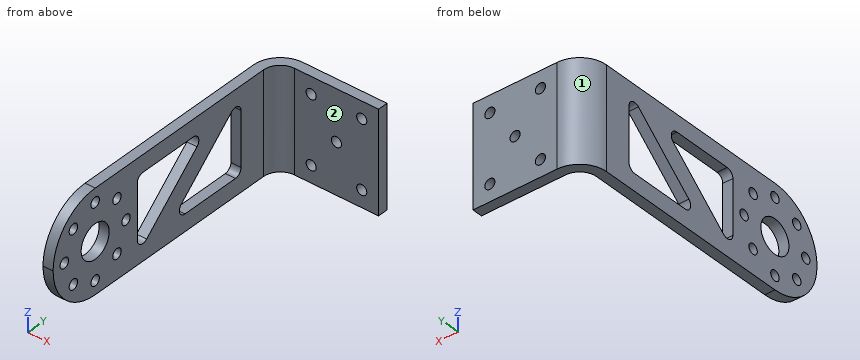
```python
from build123d import *

# Parameters (mm, degrees)
BASIS_BLECH1_DEPTH                   = 15
SCHNITT_LINEAR_AUSTRAGEN1_DEPTH      = 76.822160349
SCHNITT_LINEAR_AUSTRAGEN1_DEPTH_BACK = 76.822160349
SKIZZE2_R                            = 5
VERRUNDUNG1_R                        = 15
F_3_0_3_DURCHMESSER_BOHRUNG1_D       = 3
F_3_0MM_DOWEL_HOLE1_D                = 3


# Sheet-metal steps are written as plain solids
with BuildPart() as part:
    # Skizze1 → Basis-Blech1 (new, symmetric)
    with BuildSketch(Plane.XY):
        with BuildLine():
            Line((0, -15), (0, 60))
            ThreePointArc((0, 60), (1.464466094, 63.535533906), (5, 65))
            Line((5, 65), (30, 65))
            Line((30, 65), (30, 68))
            Line((30, 68), (5, 68))
            ThreePointArc((5, 68), (-0.656854249, 65.656854249), (-3, 60))
            Line((-3, 60), (-3, -15))
            Line((-3, -15), (0, -15))
        make_face()
    extrude(amount=BASIS_BLECH1_DEPTH, both=True)

    # Skizze2 → Schnitt-Linear austragen1 (cut, two sides: drawn at the far end of the back side and taken through both)
    with BuildSketch(Plane(origin=(0, 0, 0), x_dir=(0, 0, -1), z_dir=(1, 0, 0)).offset(-SCHNITT_LINEAR_AUSTRAGEN1_DEPTH_BACK)):
        Circle(SKIZZE2_R)
        with BuildLine():
            Line((-8, 52), (8, 52))
            ThreePointArc((8, 52), (9.414213562, 51.414213562), (10, 50))
            Line((10, 50), (10, 32.035443619))
            ThreePointArc((10, 32.035443619), (8.711675965, 30.166348298), (6.506482679, 30.705253403))
            Line((6.506482679, 30.705253403), (-9.493517321, 48.669809784))
            ThreePointArc((-9.493517321, 48.669809784), (-9.824880877, 50.818419076), (-8, 52))
        make_face()
        with BuildLine():
            Line((-6.506482679, 36.294746597), (9.493517321, 18.330190216))
            ThreePointArc((9.493517321, 18.330190216), (9.824880877, 16.181580924), (8, 15))
            Line((8, 15), (-8, 15))
            ThreePointArc((-8, 15), (-9.414213562, 15.585786438), (-10, 17))
            Line((-10, 17), (-10, 34.964556381))
            ThreePointArc((-10, 34.964556381), (-8.711675965, 36.833651702), (-6.506482679, 36.294746597))
        make_face()
    extrude(amount=SCHNITT_LINEAR_AUSTRAGEN1_DEPTH + SCHNITT_LINEAR_AUSTRAGEN1_DEPTH_BACK, mode=Mode.SUBTRACT)

    # Verrundung1
    verrundung1_edges = [part.edges().sort_by_distance(p)[0] for p in [
        (-1.5, -15, -15),
        (-1.5, -15, 15),
    ]]
    fillet(verrundung1_edges, radius=VERRUNDUNG1_R - 0.0001)  # a hair under: the kernel refuses the full size

    # Ø3.0 (3) Durchmesser Bohrung1 (through all)
    with Locations(Plane(origin=(0, 0, 0), x_dir=(0, 0, -1), z_dir=(1, 0, 0))):
        with Locations((11, 0), (7.778174593, 7.778174593), (0, 11), (-7.778174593, 7.778174593), (-11, 0), (-7.778174593, -7.778174593), (0, -11), (7.778174593, -7.778174593)):
            Hole(F_3_0_3_DURCHMESSER_BOHRUNG1_D / 2)

    # Ø3.0mm Dowel Hole1 (through all)
    with Locations(Plane(origin=(0, 68, 0), x_dir=(1, 0, 0), z_dir=(0, 1, 0))):
        with Locations((10, 10), (25, 10), (17.5, 0), (10, -10), (25, -10)):
            Hole(F_3_0MM_DOWEL_HOLE1_D / 2)


solid = part.part
```
Design review of the part built by this model. Coordinates are the model's own, in mm. Face numbers are marked on the shaded views. A direction names the side the tool comes from. Give positions to 0.01 mm unless a question says otherwise; leave off trailing zeros. Write each loop counter-clockwise with the first axis right and the second up, starting at its lowest first coordinate (ties: lowest second). Pieces come first, ordered by that corner, then holes. Notation, with made-up numbers: (86.25, 74.5) - (136.25, 74.5) arc R24 cw to (136.25, 96.5) - close; hole circle Ø5 at (61.25, 14.25). An arc over 180 degrees is marked (long way). Return JSON: item names as keys, results as strings. Group by question number.
(1) We need section D-D, the plane x = 7. Give the boundary of the cut face in (y, z).
(2) Machinability: for the marked faces 1 and 2, which of the approach directions +Z, -Z, +X, -X, +Y, -Y give a long, thin tool a straight path to every point of the face, cutting with its end or side? Answer none if there is none.
(3) To check wall thickness, follow probe 1 along Z at (x, y) = (10, 67.3); probe 2 along X at (y, z) = (66.75, 10); probe 3 along Y at (x, z) = (7, 0). State the ranges of each line that lie inside material, in increasing order.
(4) We need section C-C, the plane y = 11. Give the boundary of the cut face in (x, z), then the cut area to 3 significant figures.
(5) We need section B-B, the plane x = 17.5. Give the boundary of the cut face in (y, z).
(6) Insertion check: pin 1 (2.5 mm diameter, centred on x = 10, z = -10, fed in from -Y); pin 2 (6 mm diameter, centred on x = 16.5, z = 2, fed in from -Y); pin 3 (3.5 mm diameter, centred on x = -1, z = 3, fed in from +Y); pin 4 (4 mm diameter, centred on y = 0, z = 11, fed in from +X). Each pin has a flat end and moves straight along its axis. Give the tip position at first contact, or say it passes through.
(7) We need section A-A, the plane x = 25. Give the boundary of the cut face in (y, z).
Reported:
{
 "1": {"outline": "(65, -15) - (68, -15) - (68, 15) - (65, 15) - close"},
 "2": {"face 1": "+Z, -Z, -X, +Y", "face 2": "+Z, -Z, +X, -Y"},
 "3": {"probe 1": "z = -15 to -11.5, -8.5 to 8.5, 11.5 to 15", "probe 2": "x = 0.71 to 8.5, 11.5 to 23.5, 26.5 to 30", "probe 3": "y = 65 to 68"},
 "4": {"outline": "(-3, -15) - (0, -15) - (0, -1.5) - (-3, -1.5) - close; (-3, 1.5) - (0, 1.5) - (0, 15) - (-3, 15) - close", "area": "81.0 mm2"},
 "5": {"outline": "(65, -15) - (68, -15) - (68, -1.5) - (65, -1.5) - close; (65, 1.5) - (68, 1.5) - (68, 15) - (65, 15) - close"},
 "6": {"pin 1": "passes through", "pin 2": "stops at y = 65", "pin 3": "stops at y = 66.78", "pin 4": "stops at x = 0"},
 "7": {"outline": "(65, -15) - (68, -15) - (68, -11.5) - (65, -11.5) - close; (65, -8.5) - (68, -8.5) - (68, 8.5) - (65, 8.5) - close; (65, 11.5) - (68, 11.5) - (68, 15) - (65, 15) - close"}
}
